Could you check a few things on this model? Use its own coordinates, in mm. A direction names the side the tool comes from. Coordinates: 2 decimals unless noted, no trailing zeros. Loops run counter-clockwise (first coordinate to the right, second up) from the corner with the lowest first, then second, coordinate; pieces in that order, holes last.
1) Imagine slicing it at B-B on z = 1. Please give me the cut outline in (x, y), plus the area to 3 significant figures.
2) Imagine slicing it at D-D on y = 36. Please give me the cut outline in (x, z), plus the area to 3 significant figures.
3) If I drill on line 1 along X through (y, z) = (11, 1.4); line 2 along Y through (x, z) = (10, 1.3); line 3 along X through (y, z) = (38, 1.05), over which ranges is the centre line in solid material (lowest first)?
4) For faces 1 (the face through (17.5, 8, 1)), 2 (the face through (0, 23, 1)), which set-ups out of +Z, -Z, +X, -X, +Y, -Y let a thin tool reach every point of the face, with its end or its side?
5) Imagine slicing it at A-A on x = 30. Please give me the cut outline in (y, z).
6) Will this pin go through, and if not, where does the flat tip stop? P1, Ø3.5, axis at x = 10, y = 36, coming from the -Z side.
7) Imagine slicing it at C-C on y = 9.5. Please give me the cut outline in (x, z).
Autodesk Inventor part; units mm, degrees
ref_plane "YZ Plane" through (0, 0, 0) normal (1, 0, 0) x (0, 1, 0)
ref_plane "XZ Plane" through (0, 0, 0) normal (0, 1, 0) x (-1, 0, 0)
ref_plane "XY Plane" through (0, 0, 0) normal (0, 0, 1) x (1, 0, 0)
sketch "Sketch1" plane through (0, 0, 0) normal (0, 0, 1) x (1, 0, 0)
  line L0 (0, 0) -> (40, 0)
  line L1 (40, 0) -> (40, 46)
  line L2 (40, 46) -> (0, 46)
  line L3 (0, 46) -> (0, 0)
  line L4 (20, 0) -> (20, 15) construction
  line L5 (20, 15) -> (22.5, 15)
  line L6 (22.5, 15) -> (22.5, 0)
  line L7 (20, 15) -> (17.5, 15)
  line L8 (17.5, 15) -> (17.5, 0)
  line L9 (0, 46) -> (0, 36) construction
  line L10 (0, 36) -> (10, 36) construction
  circle A0 centre (10, 36) radius 2.75
  line L11 (40, 36) -> (30, 36) construction
  circle A1 centre (30, 36) radius 2.75
  dimension "d0" = 40
  dimension "d1" = 46
  dimension "d2" = 15
  dimension "d3" = 2.5
  dimension "d4" = 2.5
  dimension "d5" = 10
  dimension "d6" = 10
  dimension "d7" = 5.5
  dimension "d8" = 10
  dimension "d9" = 5.5
extrude "Extrusion1" add sketch "Sketch1" along normal blind 3 contours L3 L2 L1 L0 L6 L5 L7 L8
properties part number "Camera_Mount"
Filled in:
1. outline: (0, 0) - (17.5, 0) - (17.5, 15) - (22.5, 15) - (22.5, 0) - (40, 0) - (40, 46) - (0, 46) - close; hole circle Ø5.5 at (10, 36); hole circle Ø5.5 at (30, 36)
1. area: 1,720 mm2
2. outline: (0, 0) - (7.25, 0) - (7.25, 3) - (0, 3) - close; (12.75, 0) - (27.25, 0) - (27.25, 3) - (12.75, 3) - close; (32.75, 0) - (40, 0) - (40, 3) - (32.75, 3) - close
2. area: 87.0 mm2
3. line 1: x = 0 to 17.5, 22.5 to 40
3. line 2: y = 0 to 33.25, 38.75 to 46
3. line 3: x = 0 to 8.11, 11.89 to 28.11, 31.89 to 40
4. face 1: +Z, -Z, -Y
4. face 2: +Z, -Z, -X, +Y, -Y
5. outline: (0, 0) - (33.25, 0) - (33.25, 3) - (0, 3) - close; (38.75, 0) - (46, 0) - (46, 3) - (38.75, 3) - close
6. P1: passes through
7. outline: (0, 0) - (17.5, 0) - (17.5, 3) - (0, 3) - close; (22.5, 0) - (40, 0) - (40, 3) - (22.5, 3) - close
